Verification items for the finished model (mm, model axes). Face numbers are marked on the shaded views. A direction names the side the tool comes from. Coordinates: 2 decimals unless noted, no trailing zeros. Loops run counter-clockwise (first coordinate to the right, second up) from the corner with the lowest first, then second, coordinate; pieces in that order, holes last. Notation, with made-up numbers: (8, 51.5) - (29, 51.5) arc R26 ccw to (29, 81.5) - close; hole circle Ø1 at (-38, -23). An arc over 180 degrees is marked (long way). Answer as CSV lines item,"result". Start each with the question number.
1. Cross-section at C-C (y = -3.5). Enter the section's corners in (x, z).
2. Release check for a two-part mould opening along Z. For the marked faces 1, 2 and 3 record: pulls with the +Z half, pulls with the -Z half, needs draft (parallel to the pull), parting line crosses it, or undercut.
3. Set-up check for the marked faces 4 and 5: record each of +Z, -Z, +X, -X, +Y, -Y from which the full face is reachable in a straight line by a thin tool's end or side.
4. Cross-section at A-A (x = 0). Enter the section's corners in (y, z), plus the area to 3 significant figures.
5. Gauge pin test, flat ends, axial feed: P1, Ø6.5, axis at y = -9.525, z = -13.462, coming from the +X side; P2, Ø1.5, axis at y = -15, z = 1, coming from the -X side; P3, Ø2, axis at x = -4.5, y = -14.5, coming from the +Z side. Record the tip position at first contact, or that the pin passes through.
6. Cross-section at B-B (z = -6.75). Enter the section's corners in (x, y), plus the area to 3 significant figures.
7. Material ranges on line 1 (X direction, y = -0.75, z = -11.25); line 2 (Z direction, x = 4.25, y = -17); line 3 (Z direction, x = -2.75, y = -5.5), recorded low to high. Write a range as [from, to].
8. Cross-section at D-D (x = 3). State how many separate pieces and enclosed holes the cut face has, plus the area to 3 significant figures.
```python
from build123d import *

# Parameters (mm, degrees)
F1_DEPTH = 19.05
F2_SIZE  = 0.508
F4_DEPTH = 1.524
F6_D     = 4.0386
F6_DEPTH = 5.93725
F6_TIP   = 1.213317848


with BuildPart() as f1:
    # F0 (on Front) → F1 (new body)
    with BuildSketch(Plane.XZ):
        with BuildLine():
            Line((8.001, -19.812), (8.001, 0))
            ThreePointArc((8.001, 0), (0, 8.001), (-8.001, 0))
            Line((-8.001, 0), (-8.001, -19.812))
            Line((-8.001, -19.812), (-0.762, -19.812))
            Line((-0.762, -19.812), (-0.762, -5.5675371219))
            ThreePointArc((-0.762, -5.5675371219), (0, 5.6194406842), (0.762, -5.5675371219))
            Line((0.762, -5.5675371219), (0.762, -19.812))
            Line((0.762, -19.812), (8.001, -19.812))
        make_face()
    extrude(amount=F1_DEPTH)

    # F2
    f2_edges = [f1.edges().sort_by_distance(p)[0] for p in [
        (0, -19.05, 5.619441),
    ]]
    chamfer(f2_edges, length=F2_SIZE)

    # F3 (on face) → F4 (cut)
    with BuildSketch(Plane.YZ.offset(8.001)):
        with BuildLine():
            Line((0, -19.812), (0, -8.2424463785))
            ThreePointArc((0, -8.2424463785), (-9.525, -4.826), (-19.05, -8.2424463785))
            Line((-19.05, -8.2424463785), (-19.05, -19.812))
            Line((-19.05, -19.812), (0, -19.812))
        make_face()
    extrude(amount=-F4_DEPTH, mode=Mode.SUBTRACT)

    # F6
    with Locations(Plane.YZ.offset(6.477)):
        with Locations((-9.525, -13.462)):
            Hole(F6_D / 2, depth=F6_DEPTH)
            with Locations((0, 0, -(F6_DEPTH + F6_TIP / 2))):  # 118° drill point
                Cone(0, F6_D / 2, F6_TIP, mode=Mode.SUBTRACT)


solid = f1.part
```
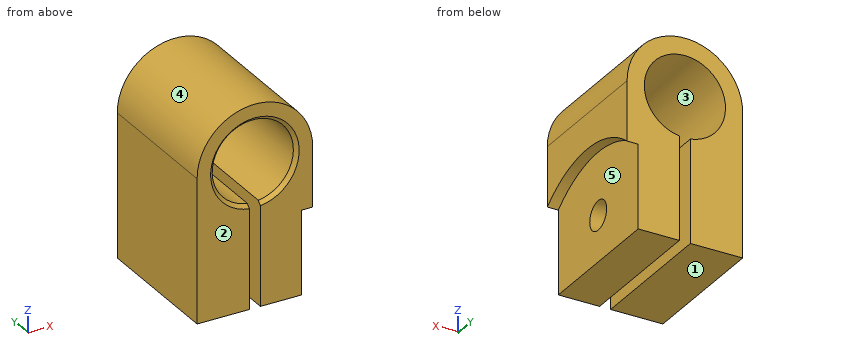
Values follow:
1,outline,"(-8, -19.81) - (-0.76, -19.81) - (-0.76, -5.57) arc R5.62 cw (long way) to (0.76, -5.57) - (0.76, -19.81) - (6.48, -19.81) - (6.48, -6.09) - (8, -6.09) - (8, 0) arc R8 ccw to (-8, 0) - close"
2,face 1,"pulls with the -Z half"
2,face 2,"needs draft"
2,face 3,"undercut"
3,face 4,"+Z, +Y, -Y"
3,face 5,"-Z, +X"
4,outline,"(-19.05, 6.13) - (-18.54, 5.62) - (0, 5.62) - (0, 8) - (-19.05, 8) - close"
4,area,"45.2 mm²"
5,P1,"stops at x = 6.48"
5,P2,"stops at x = -8"
5,P3,"stops at z = 7.19"
6,outline,"(-8, -19.05) - (-0.76, -19.05) - (-0.76, 0) - (-8, 0) - close; (0.76, -19.05) - (8, -19.05) - (8, -16.87) - (6.48, -16.87) - (6.48, -2.18) - (8, -2.18) - (8, 0) - (0.76, 0) - close"
6,area,"253 mm²"
7,line 1,"x = [-8, -0.76], [0.76, 6.48]"
7,line 2,"z = [-19.81, -3.68], [3.68, 6.78]"
7,line 3,"z = [-19.81, -4.9], [4.9, 7.51]"
8,separate pieces,"2"
8,enclosed holes,"1"
8,area,"325 mm²"
